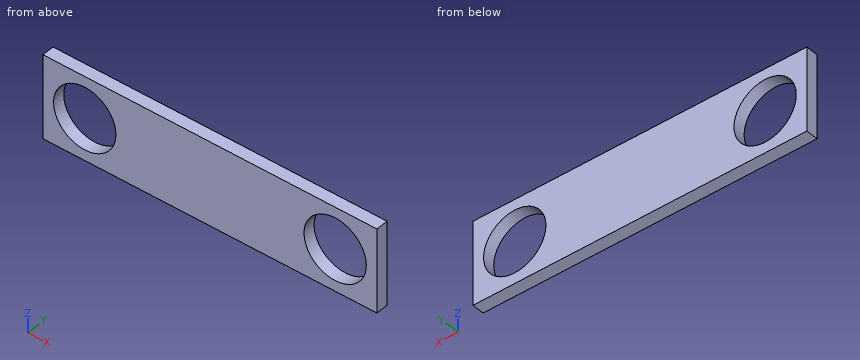
from build123d import *

# Parameters (mm, degrees)
SKETCH1_W           = 152.4
SKETCH1_H           = 38.1
BOSS_EXTRUDE1_DEPTH = 5.588
SKETCH6_R           = 14.224
CUT_EXTRUDE4_DEPTH  = 6.588
SKETCH7_R           = 14.224
CUT_EXTRUDE5_DEPTH  = 6.588


with BuildPart() as part:
    # Sketch1 → Boss-Extrude1 (new body)
    with BuildSketch(Plane(origin=(0, 0, 0), x_dir=(1, 0, 0), z_dir=(0, 1, 0))):
        with Locations((76.2, 19.05)):
            Rectangle(SKETCH1_W, SKETCH1_H)
    extrude(amount=BOSS_EXTRUDE1_DEPTH)

    # Sketch6 → Cut-Extrude4 (cut, through all)
    with BuildSketch(Plane(origin=(0, 5.588, 0), x_dir=(1, 0, 0), z_dir=(0, 1, 0))):
        with Locations((19.05, 19.05)):
            Circle(SKETCH6_R)
    extrude(amount=-CUT_EXTRUDE4_DEPTH, mode=Mode.SUBTRACT)

    # Sketch7 → Cut-Extrude5 (cut, through all)
    with BuildSketch(Plane(origin=(0, 5.588, 0), x_dir=(1, 0, 0), z_dir=(0, 1, 0))):
        with Locations((133.35, 19.05)):
            Circle(SKETCH7_R)
    extrude(amount=-CUT_EXTRUDE5_DEPTH, mode=Mode.SUBTRACT)


solid = part.part
Source: CAD feature listing. Evaluate the final solid. Frame: model axes, mm. Give positions to 0.01 mm unless a question says otherwise; leave off trailing zeros. Order: outer loops, then holes, each group sorted by start corner. A loop starts at its lowest first (then second) coordinate and runs counter-clockwise, first axis right, second up. Notation, with made-up numbers: (-13.5, 80) -> (45.5, 80) arc R15 ccw to (45.5, 93) -> close; hole circle Ø5 at (88, 75.25). An arc over 180 degrees is marked (long way). Write item = value, one per line.
Q1. Cut plane D-D, the plane z = -7.5. Output: boundary loops of the cut face in (x, y), and give its area (3 significant figures).
Data:
outline = (0, 0) -> (10.75, 0) -> (10.75, 5.59) -> (0, 5.59) -> close; (27.35, 0) -> (125.05, 0) -> (125.05, 5.59) -> (27.35, 5.59) -> close; (141.65, 0) -> (152.4, 0) -> (152.4, 5.59) -> (141.65, 5.59) -> close
area = 666 mm^2
Q2. Cut plane A-A, the plane z = -19.05. Output: boundary loops of the cut face in (x, y).
Data:
outline = (0, 0) -> (4.83, 0) -> (4.83, 5.59) -> (0, 5.59) -> close; (33.27, 0) -> (119.13, 0) -> (119.13, 5.59) -> (33.27, 5.59) -> close; (147.57, 0) -> (152.4, 0) -> (152.4, 5.59) -> (147.57, 5.59) -> close
Q3. Cut plane B-B, the plane x = 133.35. Output: boundary loops of the cut face in (y, z), and give its area (3 significant figures).
Data:
outline = (0, -38.1) -> (5.59, -38.1) -> (5.59, -33.27) -> (0, -33.27) -> close; (0, -4.83) -> (5.59, -4.83) -> (5.59, 0) -> (0, 0) -> close
area = 53.9 mm^2
Q4. Material intervals for line 1 (X direction, y = 1.25, z = -19.05); line 2 (X direction, y = 2.7, z = -26); line 3 (Z direction, x = 133.35, y = 1.65), sorted ascending. Write a range as from..to.
Data:
line_1 = 0..4.83, 33.27..119.13, 147.57..152.4
line_2 = 0..6.64, 31.46..120.94, 145.76..152.4
line_3 = -38.1..-33.27, -4.83..0
Q5. Cut plane C-C, the plane y = 1.9. Output: boundary loops of the cut face in (x, z).
Data:
outline = (0, -38.1) -> (152.4, -38.1) -> (152.4, 0) -> (0, 0) -> close; hole circle Ø28.45 at (19.05, -19.05); hole circle Ø28.45 at (133.35, -19.05)
